The listing builds one solid part. Answer for the finished solid, in the listing's coordinates (mm). Face numbers are marked on the shaded views. A direction names the side the tool comes from. Coordinates: 2 decimals unless noted, no trailing zeros. Order: outer loops, then holes, each group sorted by start corner. A loop starts at its lowest first (then second) coordinate and runs counter-clockwise, first axis right, second up. Notation, with made-up numbers: (6, -14.75) -> (45, -14.75) arc R38 ccw to (45, 24.25) -> close; hole circle Ø2 at (-2, 26.25). An arc over 180 degrees is marked (long way). One line per question, with ' | ' between items.
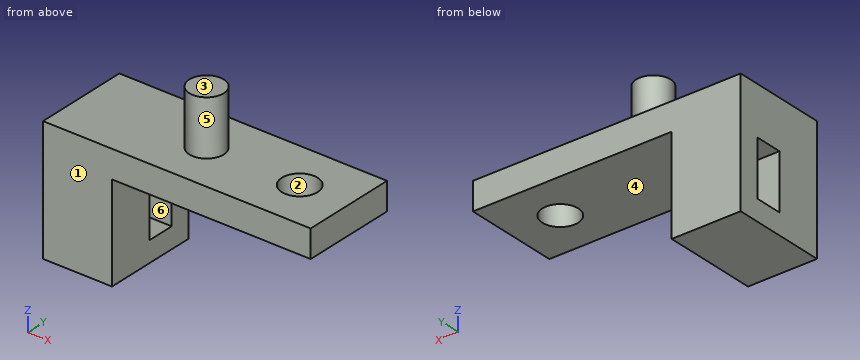
from build123d import *

# Parameters (mm, degrees)
BOSS_EXTRUDE1_DEPTH = 6.9
SKETCH2_R           = 1.3
CUT_EXTRUDE1_DEPTH  = 10
SKETCH3_R           = 1.25
BOSS_EXTRUDE2_DEPTH = 4
SKETCH4_W           = 4
SKETCH4_H           = 2
CUT_EXTRUDE2_DEPTH  = 6


with BuildPart() as part:
    # Sketch1 → Boss-Extrude1 (new body)
    with BuildSketch(Plane(origin=(0, 0, 0), x_dir=(1, 0, 0), z_dir=(0, 1, 0))):
        Polygon((154.749006664, -21.005499154), (135.349006664, -21.005499154), (135.349006664, -12.005499154), (140.349006664, -12.005499154), (140.349006664, -19.005499154), (154.749006664, -19.005499154), align=None)
    extrude(amount=BOSS_EXTRUDE1_DEPTH)

    # Sketch2 → Cut-Extrude1 (cut, through all)
    with BuildSketch(Plane.XY.offset(21.005499154)):
        with Locations((151.189006664, 3.45)):
            Circle(SKETCH2_R)
    extrude(amount=-CUT_EXTRUDE1_DEPTH, mode=Mode.SUBTRACT)

    # Sketch3 → Boss-Extrude2 (add)
    with BuildSketch(Plane.XY.offset(21.005499154)):
        with Locations((144.439006664, 3.45)):
            Circle(SKETCH3_R)
    extrude(amount=BOSS_EXTRUDE2_DEPTH)

    # Sketch4 → Cut-Extrude2 (cut, through all)
    with BuildSketch(Plane(origin=(140.349006664, 0, 0), x_dir=(0, 0, -1), z_dir=(1, 0, 0))):
        with Locations((-15.505499154, 4.4)):
            Rectangle(SKETCH4_W, SKETCH4_H)
    extrude(amount=-CUT_EXTRUDE2_DEPTH, mode=Mode.SUBTRACT)


solid = part.part
Item 1: For the marked faces 4, 5 and 6, determine the directions among +Z, -Z, +X, -X, +Y, -Y from which every point of the face is accessible in a straight line to the end or side of a thin tool.
Computed values:
face 4: -Z, +X, +Y, -Y | face 5: +Z | face 6: +X, -X
Item 2: Determine the mould class of the marked faces 1, 2 and 3 for opening direction Y: pulls with the +Y half, pulls with the -Y half, needs draft (parallel to the pull), parting line crosses it, or undercut.
Computed values:
face 1: pulls with the -Y half | face 2: undercut | face 3: needs draft
Item 3: Each of these flat-tipped pins is pushed along its axis until it touches: pin 1 Ø2 at (x, y) = (137, 5) entering from +Z; pin 2 Ø3 at (y, z) = (4.5, 16) entering from +X; pin 3 Ø1 at (x, y) = (149.5, 2.5) entering from -Z. Where does it stop, or does it pass through?
Computed values:
pin 1: stops at z = 21.01 | pin 2: stops at x = 140.35 | pin 3: stops at z = 19.01
Item 4: Section D-D, the plane y = 4.5 is taken. Give the vertices of the cut face in (x, z).
Computed values:
outline: (135.35, 12.01) -> (140.35, 12.01) -> (140.35, 13.51) -> (135.35, 13.51) -> close; (135.35, 17.51) -> (140.35, 17.51) -> (140.35, 19.01) -> (150.42, 19.01) -> (150.42, 21.01) -> (145.12, 21.01) -> (145.12, 25.01) -> (143.76, 25.01) -> (143.76, 21.01) -> (135.35, 21.01) -> close; (151.96, 19.01) -> (154.75, 19.01) -> (154.75, 21.01) -> (151.96, 21.01) -> close
Item 5: Find the intervals of material crossed by L1, parallel to Y at x = 136.5, z = 14.75; L2, parallel to X at y = 6.5, z = 18; L3, parallel to Z at x = 154, y = 2, in increasing order.
Computed values:
L1: y = 0 to 3.4, 5.4 to 6.9 | L2: x = 135.35 to 140.35 | L3: z = 19.01 to 21.01
Item 6: Section B-B, the plane x = 138.25 is taken. Give the vertices of the cut face in (y, z).
Computed values:
outline: (0, 12.01) -> (6.9, 12.01) -> (6.9, 21.01) -> (0, 21.01) -> close; hole (3.4, 13.51) -> (5.4, 13.51) -> (5.4, 17.51) -> (3.4, 17.51) -> close
Item 7: Section C-C, the plane x = 151.75 is taken. Give the vertices of the cut face in (y, z), plus the area to 3 significant figures.
Computed values:
outline: (0, 19.01) -> (2.28, 19.01) -> (2.28, 21.01) -> (0, 21.01) -> close; (4.62, 19.01) -> (6.9, 19.01) -> (6.9, 21.01) -> (4.62, 21.01) -> close | area: 9.11 mm^2
Item 8: Section A-A, the plane y = 2.5 is taken. Give the vertices of the cut face in (x, z), plus the area to 3 significant figures.
Computed values:
outline: (135.35, 12.01) -> (140.35, 12.01) -> (140.35, 19.01) -> (150.3, 19.01) -> (150.3, 21.01) -> (145.25, 21.01) -> (145.25, 25.01) -> (143.63, 25.01) -> (143.63, 21.01) -> (135.35, 21.01) -> close; (152.08, 19.01) -> (154.75, 19.01) -> (154.75, 21.01) -> (152.08, 21.01) -> close | area: 76.7 mm^2
